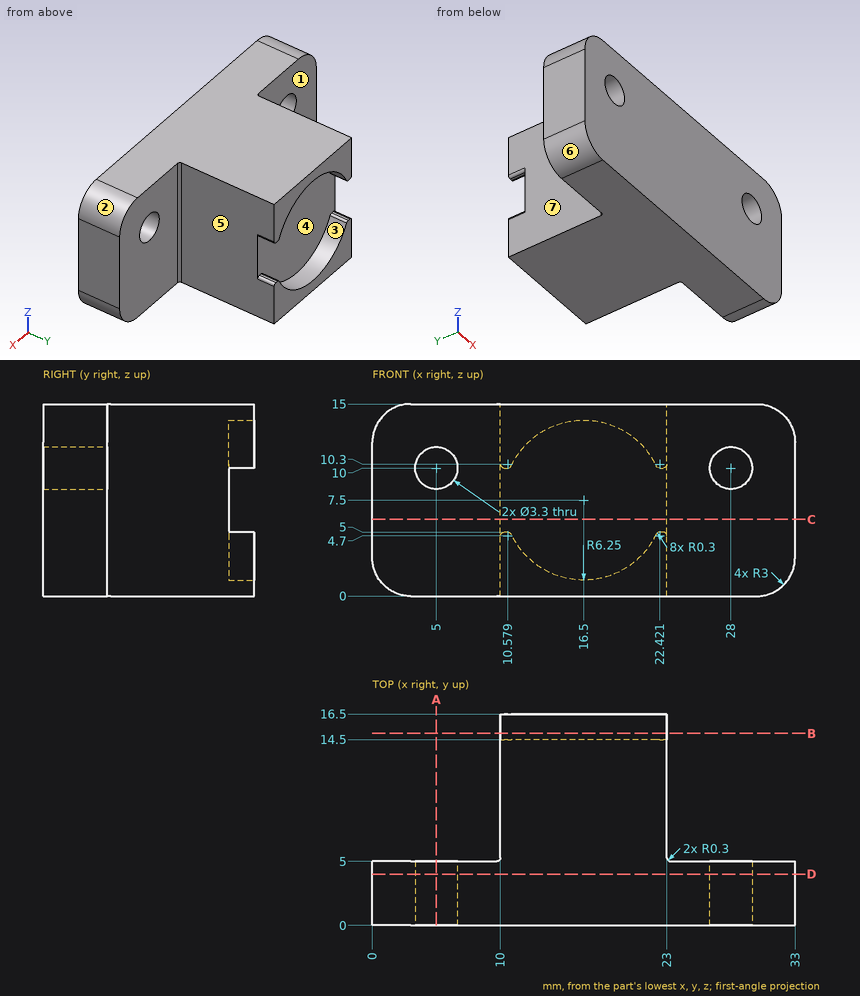
Design review of the part shown in the three views and the two pictorial views. Dimensions are in mm from the part's minimum x, y and z. A direction names the side the tool comes from. Coordinates: 2 decimals unless noted, no trailing zeros. Order: outer loops, then holes, each group sorted by start corner. A loop starts at its lowest first (then second) coordinate and runs counter-clockwise, first axis right, second up. Notation, with made-up numbers: (-14.75, -11) - (16.25, -11) arc R17 cw to (16.25, 5) - close; hole circle Ø11 at (45, 78.5). An arc over 180 degrees is marked (long way). Answer as CSV lines item,"result". Start each with the question number.
1) To check wall thickness, follow line 1 along Z through (x, y) = (5, 2.55); line 2 along X through (y, z) = (9.25, 12.25); line 3 along Y through (x, z) = (31, 2.5). State the ranges of each line that lie inside material, in increasing order. Write a range as [from, to].
2) Add section A-A (x = 5). State the section outline as (y, z) points, then the cut area to 3 significant figures.
3) Insertion check: P1, Ø3.5, axis at y = 9, z = 4.5, coming from the +X side; P2, Ø8, axis at x = 28.5, z = 11, coming from the +Y side; P3, Ø3, axis at y = 7.5, z = 2.5, coming from the -X side. Each pin has a flat end and moves straight along its axis. Give the tip position at first contact, or say it passes through.
4) Draft analysis for pull direction X (two halves, no side actions). For the marked faces 1, 2, 3 and 4, state which applies: +X half, -X half, draft (parallel to the pull), parting line (faces both ways), or undercut.
5) Add section B-B (y = 15). State the section outline as (x, z) points.
6) Add section D-D (y = 4). State the section outline as (x, z) points.
7) Add section C-C (z = 6). State the section outline as (x, y) points.
8) Machinability: for the marked faces 5, 6 and 7, which of the approach directions +Z, -Z, +X, -X, +Y, -Y give a long, thin tool a straight path to every point of the face, cutting with its end or side? Answer none if there is none.
Result:
1,line 1,"[0, 8.35], [11.65, 15]"
1,line 2,"[10, 23]"
1,line 3,"[0, 5]"
2,outline,"(0, 0) - (5, 0) - (5, 8.35) - (0, 8.35) - close; (0, 11.65) - (5, 11.65) - (5, 15) - (0, 15) - close"
2,area,"58.5 mm^2"
3,P1,"x = 23"
3,P2,"y = 5"
3,P3,"x = 10"
4,face 1,"draft"
4,face 2,"+X half"
4,face 3,"undercut"
4,face 4,"undercut"
5,outline,"(10, 0) - (23, 0) - (23, 4.7) arc R0.3 ccw to (22.7, 5) - (22.42, 5) arc R0.3 ccw to (22.15, 4.83) arc R6.25 cw to (10.85, 4.83) arc R0.3 ccw to (10.58, 5) - (10.3, 5) arc R0.3 ccw to (10, 4.7) - close; (10, 10.3) arc R0.3 ccw to (10.3, 10) - (10.58, 10) arc R0.3 ccw to (10.85, 10.17) arc R6.25 cw to (22.15, 10.17) arc R0.3 ccw to (22.42, 10) - (22.7, 10) arc R0.3 ccw to (23, 10.3) - (23, 15) - (10, 15) - close"
6,outline,"(0, 3) arc R3 ccw to (3, 0) - (30, 0) arc R3 ccw to (33, 3) - (33, 12) arc R3 ccw to (30, 15) - (3, 15) arc R3 ccw to (0, 12) - close; hole circle Ø3.3 at (5, 10); hole circle Ø3.3 at (28, 10)"
7,outline,"(0, 0) - (33, 0) - (33, 5) - (23.3, 5) arc R0.3 cw to (23, 5.3) - (23, 14.5) - (10, 14.5) - (10, 5.3) arc R0.3 cw to (9.7, 5) - (0, 5) - close"
8,face 5,"+Z, -Z, +X, +Y"
8,face 6,"-Z, -X, +Y, -Y"
8,face 7,"+Z, -Z, -X, +Y"
